```python
from build123d import *

# Parameters (mm, degrees)
F0_R     = 63.5
F0_R_2   = 50.8
F1_DEPTH = 88.9
F4_DEPTH = 76.2


# Not quite as in the source:
# - a feature of the source that left no trace in its solid (it failed there, or was rolled back) is left out


with BuildPart() as f1:
    # F0 (on Top) → F1 (new body)
    with BuildSketch(Plane.XY):
        Circle(F0_R)
        Circle(F0_R_2, mode=Mode.SUBTRACT)
    extrude(amount=F1_DEPTH)

    # F3 (on face) → F4 (cut)
    with BuildSketch(Plane.XY.offset(88.9)):
        with BuildLine():
            Line((-1.905, -6.8671500075), (-1.905, -3.0571500075))
            Line((-1.905, -3.0571500075), (-2.6940768363, -2.2680731712))
            Line((-2.6940768363, -2.2680731712), (-36.1333947901, -35.7073911249))
            ThreePointArc((-36.1333947901, -35.7073911249), (-34.768258257, -37.0379294477), (-33.3541627773, -38.3163127848))
            Line((-33.3541627773, -38.3163127848), (-1.905, -6.8671500075))
        make_face()
        with BuildLine():
            ThreePointArc((-45.1137772181, -44.6877735529), (-43.7523970967, -46.0214922432), (-42.3516057863, -47.3137557938))
            Line((-42.3516057863, -47.3137557938), (-33.3541627773, -38.3163127848))
            ThreePointArc((-33.3541627773, -38.3163127848), (-34.768258257, -37.0379294477), (-36.1333947901, -35.7073911249))
            Line((-36.1333947901, -35.7073911249), (-45.1137772181, -44.6877735529))
        make_face()
        with BuildLine():
            Line((-44.6998995402, -49.6620495477), (-42.3516057863, -47.3137557938))
            ThreePointArc((-42.3516057863, -47.3137557938), (-43.7523970967, -46.0214922432), (-45.1137772181, -44.6877735529))
            Line((-45.1137772181, -44.6877735529), (-47.3939763765, -46.9679727114))
            Line((-47.3939763765, -46.9679727114), (-44.6998995402, -49.6620495477))
        make_face()
        with BuildLine():
            Line((-67.31, -1.905), (-63.4714185677, -1.905))
            ThreePointArc((-63.4714185677, -1.905), (-63.5, 0), (-63.4714185677, 1.905))
            Line((-63.4714185677, 1.905), (-67.31, 1.905))
            Line((-67.31, 1.905), (-67.31, -1.905))
        make_face()
        with BuildLine():
            ThreePointArc((-63.4714185677, 1.905), (-63.5, 0), (-63.4714185677, -1.905))
            Line((-63.4714185677, -1.905), (-50.7642686838, -1.905))
            ThreePointArc((-50.7642686838, -1.905), (-50.8, 0), (-50.7642686838, 1.905))
            Line((-50.7642686838, 1.905), (-63.4714185677, 1.905))
        make_face()
        with BuildLine():
            Line((-50.7642686838, -1.905), (-3.0571500075, -1.905))
            Line((-3.0571500075, -1.905), (-6.8671500075, 1.905))
            Line((-6.8671500075, 1.905), (-50.7642686838, 1.905))
            ThreePointArc((-50.7642686838, 1.905), (-50.8, 0), (-50.7642686838, -1.905))
        make_face()
        with BuildLine():
            Line((-6.8671500075, 1.905), (-1.905, 1.905))
            Line((-1.905, 1.905), (-1.905, 2.3310036652))
            Line((-1.905, 2.3310036652), (-35.7073911249, 36.1333947901))
            ThreePointArc((-35.7073911249, 36.1333947901), (-37.0379294477, 34.768258257), (-38.3163127848, 33.3541627773))
            Line((-38.3163127848, 33.3541627773), (-6.8671500075, 1.905))
        make_face()
        with BuildLine():
            Line((1.905, 1.905), (6.8671500075, 1.905))
            Line((6.8671500075, 1.905), (38.3163127848, 33.3541627773))
            ThreePointArc((38.3163127848, 33.3541627773), (37.0379294477, 34.768258257), (35.7073911249, 36.1333947901))
            Line((35.7073911249, 36.1333947901), (1.905, 2.3310036652))
            Line((1.905, 2.3310036652), (1.905, 1.905))
        make_face()
        with BuildLine():
            Line((3.0571500075, -1.905), (50.7642686838, -1.905))
            ThreePointArc((50.7642686838, -1.905), (50.7910663854, -0.9526675347), (50.8, 0))
            ThreePointArc((50.8, 0), (50.7910663854, 0.9526675347), (50.7642686838, 1.905))
            Line((50.7642686838, 1.905), (6.8671500075, 1.905))
            Line((6.8671500075, 1.905), (3.0571500075, -1.905))
        make_face()
        with BuildLine():
            Line((50.7642686838, -1.905), (63.4714185677, -1.905))
            ThreePointArc((63.4714185677, -1.905), (63.4928542399, -0.9526071985), (63.5, 0))
            ThreePointArc((63.5, 0), (63.4928542399, 0.9526071985), (63.4714185677, 1.905))
            Line((63.4714185677, 1.905), (50.7642686838, 1.905))
            ThreePointArc((50.7642686838, 1.905), (50.7910663854, 0.9526675347), (50.8, 0))
            ThreePointArc((50.8, 0), (50.7910663854, -0.9526675347), (50.7642686838, -1.905))
        make_face()
        with BuildLine():
            Line((38.3163127848, 33.3541627773), (47.3137557938, 42.3516057863))
            ThreePointArc((47.3137557938, 42.3516057863), (46.0214922432, 43.7523970967), (44.6877735529, 45.1137772181))
            Line((44.6877735529, 45.1137772181), (35.7073911249, 36.1333947901))
            ThreePointArc((35.7073911249, 36.1333947901), (37.0379294477, 34.768258257), (38.3163127848, 33.3541627773))
        make_face()
        with BuildLine():
            ThreePointArc((33.3541627773, -38.3163127848), (34.768258257, -37.0379294477), (36.1333947901, -35.7073911249))
            Line((36.1333947901, -35.7073911249), (2.6940768363, -2.2680731712))
            Line((2.6940768363, -2.2680731712), (1.905, -3.0571500075))
            Line((1.905, -3.0571500075), (1.905, -6.8671500075))
            Line((1.905, -6.8671500075), (33.3541627773, -38.3163127848))
        make_face()
        with BuildLine():
            ThreePointArc((42.3516057863, -47.3137557938), (43.7523970967, -46.0214922432), (45.1137772181, -44.6877735529))
            Line((45.1137772181, -44.6877735529), (36.1333947901, -35.7073911249))
            ThreePointArc((36.1333947901, -35.7073911249), (34.768258257, -37.0379294477), (33.3541627773, -38.3163127848))
            Line((33.3541627773, -38.3163127848), (42.3516057863, -47.3137557938))
        make_face()
        with BuildLine():
            Line((52.015964851, -51.5899611858), (45.1137772181, -44.6877735529))
            ThreePointArc((45.1137772181, -44.6877735529), (43.7523970967, -46.0214922432), (42.3516057863, -47.3137557938))
            Line((42.3516057863, -47.3137557938), (49.3218880147, -54.2840380222))
            Line((49.3218880147, -54.2840380222), (52.015964851, -51.5899611858))
        make_face()
        with BuildLine():
            Line((63.4714185677, -1.905), (67.31, -1.905))
            Line((67.31, -1.905), (67.31, 1.905))
            Line((67.31, 1.905), (63.4714185677, 1.905))
            ThreePointArc((63.4714185677, 1.905), (63.4928542399, 0.9526071985), (63.5, 0))
            ThreePointArc((63.5, 0), (63.4928542399, -0.9526071985), (63.4714185677, -1.905))
        make_face()
        with BuildLine():
            ThreePointArc((44.6877735529, 45.1137772181), (46.0214922432, 43.7523970967), (47.3137557938, 42.3516057863))
            Line((47.3137557938, 42.3516057863), (51.0685980704, 46.106448063))
            Line((51.0685980704, 46.106448063), (48.3745212341, 48.8005248993))
            Line((48.3745212341, 48.8005248993), (44.6877735529, 45.1137772181))
        make_face()
        with BuildLine():
            Line((-35.7073911249, 36.1333947901), (-44.6877735529, 45.1137772181))
            ThreePointArc((-44.6877735529, 45.1137772181), (-46.0214922432, 43.7523970967), (-47.3137557938, 42.3516057863))
            Line((-47.3137557938, 42.3516057863), (-38.3163127848, 33.3541627773))
            ThreePointArc((-38.3163127848, 33.3541627773), (-37.0379294477, 34.768258257), (-35.7073911249, 36.1333947901))
        make_face()
        with BuildLine():
            Line((-1.4789963348, 1.905), (1.4789963348, 1.905))
            Line((1.4789963348, 1.905), (1.905, 2.3310036652))
            Line((1.905, 2.3310036652), (1.905, 50.7642686838))
            ThreePointArc((1.905, 50.7642686838), (0, 50.8), (-1.905, 50.7642686838))
            Line((-1.905, 50.7642686838), (-1.905, 2.3310036652))
            Line((-1.905, 2.3310036652), (-1.4789963348, 1.905))
        make_face()
        with BuildLine():
            Line((1.905, 50.7642686838), (1.905, 63.4714185677))
            ThreePointArc((1.905, 63.4714185677), (0, 63.5), (-1.905, 63.4714185677))
            Line((-1.905, 63.4714185677), (-1.905, 50.7642686838))
            ThreePointArc((-1.905, 50.7642686838), (0, 50.8), (1.905, 50.7642686838))
        make_face()
        with BuildLine():
            ThreePointArc((-47.3137557938, 42.3516057863), (-46.0214922432, 43.7523970967), (-44.6877735529, 45.1137772181))
            Line((-44.6877735529, 45.1137772181), (-47.5721312908, 47.998134956))
            Line((-47.5721312908, 47.998134956), (-50.2662081271, 45.3040581197))
            Line((-50.2662081271, 45.3040581197), (-47.3137557938, 42.3516057863))
        make_face()
        with BuildLine():
            ThreePointArc((-1.905, 63.4714185677), (0, 63.5), (1.905, 63.4714185677))
            Line((1.905, 63.4714185677), (1.905, 67.31))
            Line((1.905, 67.31), (-1.905, 67.31))
            Line((-1.905, 67.31), (-1.905, 63.4714185677))
        make_face()
        with BuildLine():
            ThreePointArc((-1.905, -63.4714185677), (0, -63.5), (1.905, -63.4714185677))
            Line((1.905, -63.4714185677), (1.905, -50.7642686838))
            ThreePointArc((1.905, -50.7642686838), (0, -50.8), (-1.905, -50.7642686838))
            Line((-1.905, -50.7642686838), (-1.905, -63.4714185677))
        make_face()
        with BuildLine():
            Line((1.905, -50.7642686838), (1.905, -6.8671500075))
            Line((1.905, -6.8671500075), (0, -4.9621500075))
            Line((0, -4.9621500075), (-1.905, -6.8671500075))
            Line((-1.905, -6.8671500075), (-1.905, -50.7642686838))
            ThreePointArc((-1.905, -50.7642686838), (0, -50.8), (1.905, -50.7642686838))
        make_face()
    extrude(amount=-F4_DEPTH, mode=Mode.SUBTRACT)


solid = f1.part
```
The model under review builds one solid part; all positions refer to its coordinate system, in mm. A direction names the side the tool comes from. Round coordinates to 2 decimals unless told otherwise and drop trailing zeros. Write each loop counter-clockwise with the first axis right and the second up, starting at its lowest first coordinate (ties: lowest second). Pieces come first, ordered by that corner, then holes.
(1) Mouldability with a two-part tool opening along X and no side actions: class faces 5 (the flat face through (42.75, 37.79, 51.33)), 6 (the flat face through (-57, 1.905, 51)), 7 (the flat face through (-40.135, 40.561, 51.333)) as +X half, -X half, draft (parallel to the pull), parting line (faces both ways), or undercut.
(2) Machinability: for faces 1 (the flat face through (0, 57, 12.7)), 2 (the flat face through (57, 0, 12.7)), 3 (the flat face through (-42, 39, 12.7)), 4 (the flat face through (23, 53, 88.9)), which of the approach directions +Z, -Z, +X, -X, +Y, -Y give a long, thin tool a straight path to every point of the face, cutting with its end or side? Answer none if there is none.
(3) We need section A-A on z = 28.5. Give the number of separate pieces and of enclosed holes in the cut face, and give its area (3 significant figures).
(4) We need section B-B on y = 0. Give the boundary of the cut face in (x, z).
(5) Insertion check: pin 1 (1 mm diameter, centred on y = 34.5, z = 12.5, fed in from +X); pin 2 (13 mm diameter, centred on x = 43, y = 39.5, fed in from +Z); pin 3 (4 mm diameter, centred on y = 59.5, z = 36, fed in from +X); pin 4 (6 mm diameter, centred on x = -15.5, z = 9, fed in from -Y). Each pin has a flat end and moves straight along its axis. Give the tip position at first contact, or say it passes through.
(6) Wall thickness on L1, parallel to X at y = 38, z = 27; L2, parallel to Y at x = 39, z = 45.5; L3, parallel to Y at x = -52.5, z = 85.5 (3 decimals): over which ranges is each line inside the solid? List them lowest first.
Findings below:
1. face 5: undercut
1. face 6: draft
1. face 7: undercut
2. face 1: +Z, +Y, -Y
2. face 2: +Z, +X, -X
2. face 3: +Z
2. face 4: +Z, +X, -X, +Y, -Y
3. separate pieces: 8
3. enclosed holes: 0
3. area: 4,170 mm2
4. outline: (-63.5, 0) - (-50.8, 0) - (-50.8, 12.7) - (-63.5, 12.7) - close; (50.8, 0) - (63.5, 0) - (63.5, 12.7) - (50.8, 12.7) - close
5. pin 1: stops at x = 53.63
5. pin 2: stops at z = 88.9
5. pin 3: stops at x = 26.94
5. pin 4: stops at y = -62.26
6. L1: x = -50.87 to -42.96, -37.57 to -33.71, 33.71 to 37.57, 42.96 to 50.87
6. L2: y = -50.11 to -43.96, -38.57 to -32.55, 32.55 to 34.04, 39.43 to 50.11
6. L3: y = -35.721 to -1.905, 1.905 to 35.721
